Here's how the part is built. I have some questions about the finished solid (model axes, mm). A direction names the side the tool comes from. Round coordinates to 2 decimals unless told otherwise and drop trailing zeros. Loops run counter-clockwise (first coordinate to the right, second up) from the corner with the lowest first, then second, coordinate; pieces in that order, holes last. Notation, with made-up numbers: M 78.25,42 L 87.25,42 A24 cw 87.25,64 Z; hole C -32,-4 d10. An arc over 180 degrees is marked long. Use a Markdown table: item, result.
```python
from build123d import *

# Parameters (mm, degrees)
SKETCH3_R               = 1.5
CUT_EXTRUDE1_DEPTH      = 10
MIRROR2_COPY_1_SKETCH_R = 1.5
MIRROR2_COPY_1_DEPTH    = 10
FILLET1_R               = 4
SKETCH4_W               = 23
SKETCH4_H               = 17.75
SKETCH4_R               = 1.5
CUT_EXTRUDE2_DEPTH      = 2.6
SKETCH5_W               = 33.7
SKETCH5_H               = 17.75
CUT_EXTRUDE3_DEPTH      = 0.4
BOSS_EXTRUDE1_DEPTH     = 18
SKETCH7_W               = 31
SKETCH7_H               = 54
BOSS_EXTRUDE2_DEPTH     = 2
SKETCH8_W               = 14
SKETCH8_H               = 18
CUT_EXTRUDE4_DEPTH      = 12
CUT_EXTRUDE6_START      = -12
SKETCH9_R               = 5.5
CUT_EXTRUDE6_DEPTH      = 69.462376985
CUT_EXTRUDE8_DEPTH      = 22
SKETCH11_W              = 12
SKETCH11_H              = 2
CUT_EXTRUDE9_DEPTH      = 0.4
FILLET2_R               = 2


with BuildPart() as part:
    # Sketch2 → Loft1 section 0
    with BuildSketch(Plane.XY.offset(3)):
        with BuildLine():
            Line((-42, -32), (42, -32))
            Line((42, -32), (42, 32))
            Line((42, 32), (-42, 32))
            Line((-42, 32), (-42, -32))
        make_face()
    # Sketch1 → Loft1 section 1
    with BuildSketch(Plane.XY):
        with BuildLine():
            Line((-41.75, -31.75), (41.75, -31.75))
            Line((41.75, -31.75), (41.75, 31.75))
            Line((41.75, 31.75), (-41.75, 31.75))
            Line((-41.75, 31.75), (-41.75, -31.75))
        make_face()
    loft()

    # Sketch3 → Cut-Extrude1 (cut)
    with BuildSketch(Plane(origin=(0, 0, 0), x_dir=(-1, 0, 0), z_dir=(0, 0, -1))):
        with Locations((38.767766953, -28.767766953)):
            Circle(SKETCH3_R)
    cut_extrude1 = extrude(amount=-CUT_EXTRUDE1_DEPTH, mode=Mode.SUBTRACT)

    # Mirror1: Cut-Extrude1 across plane
    add(cut_extrude1.mirror(Plane(origin=(0, 0, 0), x_dir=(0, 0, 1), z_dir=(1, 0, 0))), mode=Mode.SUBTRACT)

    # Mirror2: Cut-Extrude1 across plane
    add(cut_extrude1.mirror(Plane.ZX), mode=Mode.SUBTRACT)

    # Mirror2 copy 1 sketch → Mirror2 copy 1 (cut)
    with BuildSketch(Plane(origin=(0, 0, 0), x_dir=(1, 0, 0), z_dir=(0, 0, -1))):
        with Locations((38.767766953, -28.767766953)):
            Circle(MIRROR2_COPY_1_SKETCH_R)
    extrude(amount=-MIRROR2_COPY_1_DEPTH, mode=Mode.SUBTRACT)

    # Fillet1
    fillet1_edges = [part.edges().sort_by_distance(p)[0] for p in [
        (-41.875, 31.875, 1.5),
        (41.875, 31.875, 1.5),
        (41.875, -31.875, 1.5),
        (-41.875, -31.875, 1.5),
    ]]
    fillet(fillet1_edges, radius=FILLET1_R)

    # Sketch4 → Cut-Extrude2 (cut)
    with BuildSketch(Plane.XY.offset(3)):
        with Locations((-21, 8.875)):
            Rectangle(SKETCH4_W, SKETCH4_H)
        with Locations((-21, -8.875)):
            Rectangle(SKETCH4_W, SKETCH4_H)
        with Locations((-35.85, 15.71)):
            Circle(SKETCH4_R)
        with Locations((-6.15, -15.71)):
            Circle(SKETCH4_R)
        with Locations((-6.15, 15.71)):
            Circle(SKETCH4_R)
        with Locations(Location((-35.85, -15.71, 0), (0, 0, 180))):
            Circle(SKETCH4_R)
    extrude(amount=-CUT_EXTRUDE2_DEPTH, mode=Mode.SUBTRACT)

    # Sketch5 → Cut-Extrude3 (cut)
    with BuildSketch(Plane(origin=(0, 0, 0), x_dir=(-1, 0, 0), z_dir=(0, 0, -1))):
        with Locations((20.875, -8.875)):
            Rectangle(SKETCH5_W, SKETCH5_H)
        with Locations((20.875, 8.875)):
            Rectangle(SKETCH5_W, SKETCH5_H)
    extrude(amount=-CUT_EXTRUDE3_DEPTH, mode=Mode.SUBTRACT)

    # Sketch6 → Boss-Extrude1 (add)
    with BuildSketch(Plane(origin=(0, 0, 0), x_dir=(-1, 0, 0), z_dir=(0, 0, -1))):
        Polygon((2.684756285, -27), (2.684756285, 0), (1.184756285, 0), (1.184756285, -25), (-26.815243715, -25), (-26.815243715, 0), (-28.315243715, 0), (-28.315243715, -27), align=None)
        Polygon((2.684756285, 0), (2.684756285, 27), (-28.315243715, 27), (-28.315243715, 0), (-26.815243715, 0), (-26.815243715, 25), (1.184756285, 25), (1.184756285, 0), align=None)
    extrude(amount=BOSS_EXTRUDE1_DEPTH)

    # Sketch7 → Boss-Extrude2 (add)
    with BuildSketch(Plane(origin=(0, 0, -18), x_dir=(-1, 0, 0), z_dir=(0, 0, -1))):
        with Locations((-12.815243715, 0)):
            Rectangle(SKETCH7_W, SKETCH7_H)
    extrude(amount=BOSS_EXTRUDE2_DEPTH)

    # Sketch8 → Cut-Extrude4 (cut)
    with BuildSketch(Plane(origin=(0, 27, 0), x_dir=(1, 0, 0), z_dir=(0, 1, 0))):
        with Locations((5.815243715, 9)):
            Rectangle(SKETCH8_W, SKETCH8_H)
        with Locations((19.815243715, 9)):
            Rectangle(SKETCH8_W, SKETCH8_H)
    extrude(amount=-CUT_EXTRUDE4_DEPTH, mode=Mode.SUBTRACT)

    # Sketch9 → Cut-Extrude6 (cut)
    with BuildSketch(Plane(origin=(0, 0, 0), x_dir=(-1, 0, 0), z_dir=(0, 0, -1)).offset(CUT_EXTRUDE6_START)):
        with Locations((-33.815243715, -10)):
            Circle(SKETCH9_R)
    cut_extrude6 = extrude(amount=CUT_EXTRUDE6_DEPTH, mode=Mode.SUBTRACT)

    # Mirror3: Cut-Extrude6 across plane
    add(cut_extrude6.mirror(Plane.ZX), mode=Mode.SUBTRACT)

    # Sketch10 → Cut-Extrude8 (cut)
    with BuildSketch(Plane(origin=(0, -25, 0), x_dir=(1, 0, 0), z_dir=(0, 1, 0))):
        Polygon((15.815243715, 18), (21.815243715, 18), (21.815243715, 11), (9.815243715, 11), (9.815243715, 18), align=None)
    extrude(amount=-CUT_EXTRUDE8_DEPTH, mode=Mode.SUBTRACT)

    # Sketch11 → Cut-Extrude9 (cut)
    with BuildSketch(Plane.XY.offset(-18)):
        with Locations((15.815243715, -26)):
            Rectangle(SKETCH11_W, SKETCH11_H)
    extrude(amount=-CUT_EXTRUDE9_DEPTH, mode=Mode.SUBTRACT)

    # Fillet2
    # the kernel refuses this fillet: 2 mm, written as the material it adds along each edge
    with BuildSketch(Plane(origin=(21.815243715, -25, -11), x_dir=(0, 0, -1), z_dir=(0, -1, 0)), Plane(origin=(9.815243715, -27, -18.4), x_dir=(1, 0, 0), z_dir=(0, 1, 0))) as fillet2_piece_1:
        with BuildLine():
            CenterArc((FILLET2_R, -FILLET2_R), FILLET2_R, 90, 90)
            Line((0, -FILLET2_R), (0, 0))
            Line((0, 0), (FILLET2_R, 0))
        make_face()
    extrude(amount=2)
    with BuildSketch(Plane(origin=(9.815243715, -25, -11), x_dir=(0, 0, -1), z_dir=(0, -1, 0)), Plane(origin=(21.815243715, -25, -18.4), x_dir=(0, 0, 1), z_dir=(0, -1, 0))) as fillet2_piece_2:
        with BuildLine():
            CenterArc((FILLET2_R, FILLET2_R), FILLET2_R, 180, 90)
            Line((0, FILLET2_R), (0, 0))
            Line((0, 0), (FILLET2_R, 0))
        make_face()
    extrude(amount=2)


solid = part.part
```
Q1. I need wall thicknesses on line 1 (X direction, y = -12.5, z = -16.5); line 2 (Z direction, x = 9.5, y = -14); line 3 (Y direction, x = -6.15, z = 2.1) (3 decimals). Which ranges of each line are inside material? Lowest first, please. Write a range as from..to.
Return value:
| item | result |
|---|---|
| line 1 | x = -2.68..-1.18, 26.82..28.32 |
| line 2 | z = -20..-18, 0..3 |
| line 3 | y = -31.925..-17.21, -14.21..14.21, 17.21..31.925 |
Q2. Imagine slicing it at A-A, the plane z = -14.5. Please give me the cut outline in (x, y), then the cut area to 3 significant figures.
Return value:
| item | result |
|---|---|
| outline | M -2.68,-27 L 9.82,-27 L 9.82,-25 L -1.18,-25 L -1.18,27 L -2.68,27 Z; M 21.82,-27 L 28.32,-27 L 28.32,27 L 26.82,27 L 26.82,-25 L 21.82,-25 Z |
| area | 194 mm^2 |
Q3. Imagine slicing it at B-B, the plane x = -6.15. Give the number of separate pieces and of enclosed holes in the cut face, then the cut area to 3 significant figures.
Return value:
| item | result |
|---|---|
| separate pieces | 3 |
| enclosed holes | 0 |
| area | 161 mm^2 |
Q4. For faces 1 (the flat face through (13, 27, -19)), 2 (the cylindrical face through (21.245, -25.986, -11.601)), 3 (the flat face through (13, -27, -10)), 4 (the cylindrical face through (10.417, -26.014, -17.83)), which set-ups out of +Z, -Z, +X, -X, +Y, -Y let a thin tool reach every point of the face, with its end or its side?
Return value:
| item | result |
|---|---|
| face 1 | -Z, +X, -X, +Y |
| face 2 | +Y, -Y |
| face 3 | -Z, +X, -X, -Y |
| face 4 | -Y |
Q5. Will these pins go through, and if not, where does the flat tip stop? P1, Ø4, axis at y = 9, z = -5.5, coming from the +X side; P2, Ø8, axis at x = 17.5, z = 0.5, coming from the -Y side; P3, Ø2, axis at y = 9.5, z = -9, coming from the -X side; P4, Ø10, axis at x = 17.5, z = -15.5, coming from the +Y side.
Return value:
| item | result |
|---|---|
| P1 | stops at x = 28.32 |
| P2 | stops at y = -32 |
| P3 | stops at x = -2.68 |
| P4 | stops at y = 27 |
Q6. We'd pull the mould along X, two halves only. Please class faces 5 (the flat face through (28.315, 0, -10)), 6 (the cylindrical face through (-6.475, -17.174, 1.718)), 7 (the flat face through (13, 0, -20)): pulls with the +X half, pulls with the -X half, needs draft (parallel to the pull), parting line crosses it, or undercut.
Return value:
| item | result |
|---|---|
| face 5 | pulls with the +X half |
| face 6 | undercut |
| face 7 | needs draft |
Q7. Imagine slicing it at D-D, the plane z = -6. Please give me the cut outline in (x, y), then the cut area to 3 significant figures.
Return value:
| item | result |
|---|---|
| outline | M -2.68,-27 L 28.32,-27 L 28.32,27 L 26.82,27 L 26.82,-25 L -1.18,-25 L -1.18,27 L -2.68,27 Z |
| area | 218 mm^2 |
